Input: part model. Units: mm. Frame: model coordinates. Coordinates: 2 decimals unless noted, no trailing zeros. Write each loop counter-clockwise with the first axis right and the second up, starting at its lowest first coordinate (ties: lowest second). Pieces come first, ordered by that corner, then holes. Notation, with made-up numbers: (-31, 82) -> (13, 82) arc R7 ccw to (13, 89) -> close; hole circle Ø4 at (84, -13.5). An arc over 180 degrees is marked (long way). One line per question, with ' | ' between items. Start each with the question number.
```python
from build123d import *

# Parameters (mm, degrees)
F1_DEPTH = 8
F4_D     = 10


with BuildPart() as f1:
    # F0 (on Top) → F1 (new body)
    with BuildSketch(Plane.XY):
        Polygon((8.5, -4.907477), (8.5, 4.907477), (0, 9.814955), (-8.5, 4.907477), (-8.5, -4.907477), (0, -9.814955), align=None)
    extrude(amount=-F1_DEPTH)

    # F2 (on Right) → F3 (revolve, cut)
    with BuildSketch(Plane.YZ):
        Polygon((13.814955, 0), (8.5, 0), (13.814955, -3.06859), align=None)
    revolve(axis=Axis((0, 0, -3.475147), (0, 0, -1)), mode=Mode.SUBTRACT)

    # F4 (through all)
    with Locations(Plane.XY):
        with Locations((0, 0)):
            Hole(F4_D / 2)


solid = f1.part
```
1) First-contact query: P1, Ø9, axis at x = 0, y = 0, coming from the -Z side; P2, Ø3, axis at x = 6.5, z = -1, coming from the +Y side. Flat tips, straight axial feed; report the tip coordinate or a pass-through.
2) Ray query, line 1 (X direction, y = 3, z = -6.75); line 2 (Y direction, x = -2, z = -2.25); line 3 (Y direction, x = 0.5, z = -1.5). Return the intervals inside material, ascending.
3) Pull-direction query (X, two-part tool) for faces 1 (the face through (-4.31, -7.327, -3.944)), 2 (the face through (4.19, -7.396, -3.944)), 3 (the face through (4, -4, 0)), 4 (the face through (1.08, -4.88, -4.06)); classes: released by +X, released by -X, zero draft, split by the parting line, or undercut.
4) Section A-A, the plane z = -6. Return loops of the section in (x, y), then the cut area to 3 significant figures.
Answer block:
1) P1: passes through | P2: stops at y = 6.93
2) line 1: x = -8.5 to -4, 4 to 8.5 | line 2: y = -8.66 to -4.58, 4.58 to 8.66 | line 3: y = -9.53 to -4.97, 4.97 to 9.53
3) face 1: released by -X | face 2: released by +X | face 3: zero draft | face 4: undercut
4) outline: (-8.5, -4.91) -> (0, -9.81) -> (8.5, -4.91) -> (8.5, 4.91) -> (0, 9.81) -> (-8.5, 4.91) -> close; hole circle Ø10 at (0, 0) | area: 172 mm2
